Build history of the part. All positions in model axes, mm. Face numbers are marked on the shaded views. A direction names the side the tool comes from. Coordinates: 2 decimals unless noted, no trailing zeros. Order: outer loops, then holes, each group sorted by start corner. A loop starts at its lowest first (then second) coordinate and runs counter-clockwise, first axis right, second up. Notation, with made-up numbers: (26.5, -11) - (50.5, -11) arc R13 cw to (50.5, 4) - close; hole circle Ø4 at (24.5, 62). An arc over 180 degrees is marked (long way). Return JSON: item names as keys, results as strings.
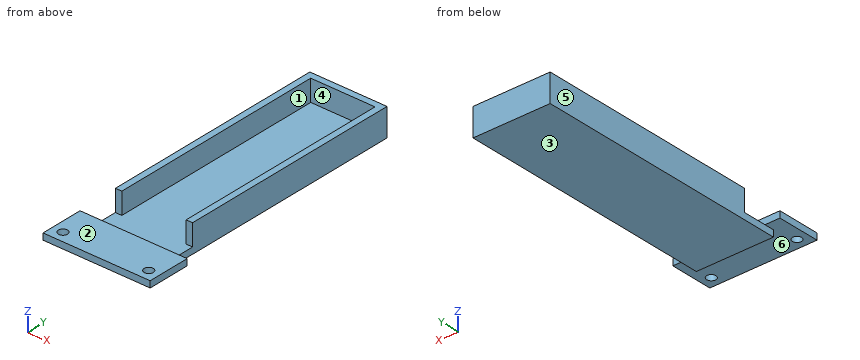
from build123d import *

# Parameters (mm, degrees)
PAD_DEPTH       = 3
PAD001_DEPTH    = 10
SKETCH002_W     = 50
SKETCH002_H     = 20
PAD002_DEPTH    = 3
SKETCH003_R     = 2.15
POCKET_DEPTH    = 5
SKETCH004_W     = 36
SKETCH004_H     = 15
POCKET001_DEPTH = 3
SKETCH005_W     = 36
SKETCH005_H     = 0.4
POCKET002_DEPTH = 3


with BuildPart() as part:
    # Sketch → Pad (new body)
    with BuildSketch(Plane.XY):
        Polygon((0, 116), (0, 0), (0, -20), (36, -20), (36, 0), (36, 116), align=None)
    extrude(amount=PAD_DEPTH)

    # Sketch001 (on Face4 of Pad) → Pad001 (join)
    with BuildSketch(Plane.XY.offset(3)):
        Polygon((0, 11), (3, 11), (3, 113), (33, 113), (33, 11), (36, 11), (36, 116), (0, 116), align=None)
    extrude(amount=PAD001_DEPTH)

    # Sketch002 (on Face3 of Pad001) → Pad002 (join)
    with BuildSketch(Plane.XY.offset(3)):
        with Locations((18, -10)):
            Rectangle(SKETCH002_W, SKETCH002_H)
    extrude(amount=PAD002_DEPTH)

    # Sketch003 (on Face13 of Pad002) → Pocket (cut)
    with BuildSketch(Plane.XY.offset(6)):
        with Locations((-2, -15)):
            Circle(SKETCH003_R)
        with Locations((38, -15)):
            Circle(SKETCH003_R)
    extrude(amount=-POCKET_DEPTH, mode=Mode.SUBTRACT)

    # Sketch004 (on Face10 of Pocket) → Pocket001 (cut)
    with BuildSketch(Plane(origin=(0, 0, 0), x_dir=(1, 0, 0), z_dir=(0, 0, -1))):
        with Locations((18, 12.5)):
            Rectangle(SKETCH004_W, SKETCH004_H)
    extrude(amount=-POCKET001_DEPTH, mode=Mode.SUBTRACT)

    # Sketch005 (on Face7 of Pocket001) → Pocket002 (cut)
    with BuildSketch(Plane(origin=(0, 0, 0), x_dir=(1, 0, 0), z_dir=(0, 0, -1))):
        with Locations((18, 4.8)):
            Rectangle(SKETCH005_W, SKETCH005_H)
    extrude(amount=-POCKET002_DEPTH, mode=Mode.SUBTRACT)


solid = part.part
1. Cut at A-A on x = -2. Give the cut face in (y, z), plus the area to 3 significant figures.
Check values:
{"outline": "(-20, 3) - (-17.15, 3) - (-17.15, 6) - (-20, 6) - close; (-12.85, 3) - (0, 3) - (0, 6) - (-12.85, 6) - close", "area": "47.1 mm²"}
2. Cut at D-D on z = 9.25. Give the cut face in (x, y), plus the area to 3 significant figures.
Check values:
{"outline": "(0, 11) - (3, 11) - (3, 113) - (33, 113) - (33, 11) - (36, 11) - (36, 116) - (0, 116) - close", "area": "720 mm²"}
3. Probe L1, parallel to Y at x = 38, z = 3.7; L2, parallel to X at y = 49.5, z = 10.75; L3, parallel to Y at x = 34, z = 3.5. List the from-to ranges inside material, lowest first.
Check values:
{"L1": "-20 to -17.15, -12.85 to 0", "L2": "0 to 3, 33 to 36", "L3": "-20 to 0, 11 to 116"}
4. Cut at C-C on y = 96. Give the cut face in (x, z), plus the area to 3 significant figures.
Check values:
{"outline": "(0, 0) - (36, 0) - (36, 13) - (33, 13) - (33, 3) - (3, 3) - (3, 13) - (0, 13) - close", "area": "168 mm²"}
5. Tool access for the marked faces 1, 2 and 3: list every direction of +Z, -Z, +X, -X, +Y, -Y with a clear straight run to the whole face (end or side of a thin tool).
Check values:
{"face 1": "+Z", "face 2": "+Z, +X, -X, -Y", "face 3": "-Z, +X, -X, +Y, -Y"}
6. Cut at B-B on y = -15. Give the cut face in (x, z).
Check values:
{"outline": "(-7, 3) - (-4.15, 3) - (-4.15, 6) - (-7, 6) - close; (0.15, 3) - (35.85, 3) - (35.85, 6) - (0.15, 6) - close; (40.15, 3) - (43, 3) - (43, 6) - (40.15, 6) - close"}
7. Drop flat-ended pins along their axis: pin 1 (6.5 mm diameter, centred on y = 50, z = 8, fed in from +X); pin 2 (6.5 mm diameter, centred on y = 65, z = 5.5, fed in from -X); pin 3 (2 mm diameter, centred on x = 35.5, z = 9.5, fed in from -Y). Give the stop position or say it passes through.
Check values:
{"pin 1": "x = 36", "pin 2": "x = 0", "pin 3": "y = 11"}
8. Mould opens along X. For the marked faces 4, 5 and 6 say: pulls with the +X half, pulls with the -X half, needs draft (parallel to the pull), parting line crosses it, or undercut.
Check values:
{"face 4": "undercut", "face 5": "pulls with the -X half", "face 6": "needs draft"}
